```python
from build123d import *

# Parameters (mm, degrees)
F0_W     = 5.75
F0_H     = 3
F2_W     = 8.114334
F2_H     = 7.330208
F3_DEPTH = 3
F4_W     = 7
F4_H     = 3
F5_DEPTH = 18.501


with BuildPart() as f1:
    # F0 (on Top) → F1 (revolve)
    with BuildSketch(Plane.XY):
        with BuildLine():
            Line((4.5, 18.5), (0, 18.5))
            Line((0, 18.5), (0, 6))
            Line((0, 6), (5.75, 6))
            Line((5.75, 6), (5.75, 8))
            add(Edge.make_bspline(
                [(5.75, 8), (5.75, 9.5), (4.5, 10), (4.5, 11.5)],
                knots=[0, 0, 0, 0, 3.716517, 3.716517, 3.716517, 3.716517], degree=3))
            Line((4.5, 11.5), (4.5, 18.5))
        make_face()
        with Locations((2.875, 1.5)):
            Rectangle(F0_W, F0_H)
    revolve(axis=Axis((0, 7.539056, 0), (0, -1, 0)))

    # F2 (on face) → F3 (join, through all)
    with BuildSketch(Plane(origin=(0, 3, 0), x_dir=(-1, 0, 0), z_dir=(0, 1, 0))):
        Rectangle(F2_W, F2_H)
    extrude(amount=F3_DEPTH)

    # F4 (on face) → F5 (cut, through all)
    with BuildSketch(Plane(origin=(0, 18.5, 0), x_dir=(-1, 0, 0), z_dir=(0, 1, 0))):
        Rectangle(F4_W, F4_H)
    extrude(amount=-F5_DEPTH, mode=Mode.SUBTRACT)


solid = f1.part
```
Check sheet for the modelled part. Datum: model origin and axes. Units: mm. A direction names the side the tool comes from. Give positions to 0.01 mm unless a question says otherwise; leave off trailing zeros. Write each loop counter-clockwise with the first axis right and the second up, starting at its lowest first coordinate (ties: lowest second). Pieces come first, ordered by that corner, then holes.
Item 1: Gauge pin test, flat ends, axial feed: pin 1 (2.5 mm diameter, centred on y = 12.5, z = -0.5, fed in from -X); pin 2 (0.9 mm diameter, centred on y = 4, z = -0.5, fed in from -X); pin 3 (5.5 mm diameter, centred on x = 1.5, y = 12.5, fed in from -Z) (3 decimals). Record the tip position at first contact, or that the pin passes through.
Item 2: Cross-section at B-B (y = 13). Enter the section's corners in (x, z).
Item 3: Access from +Z, -Z, +X, -X, +Y, -Y to the whole of each face (thin tool, end or side, straight path). Record for faces 1 (the face through (4.057, 4, 0)), 2 (the face through (-3.5, 9, 0)), 3 (the face through (-0.59, 15.05, 4.46)), 4 (the face through (-4.057, 4, 0)), 5 (the face through (0, 4, -3.665)).
Item 4: Cross-section at A-A (y = 3.5). Enter the section's corners in (x, z).
Item 5: Scan lines: L1, parallel to X at y = 5.75, z = -0.5; L2, parallel to Z at x = 2.25, y = 4; L3, parallel to Y at x = -4.25, z = -1. Record each from-to range of solid material in increasing order.
Item 6: Draft check along Z on faces 6 (the face through (0, 4, 3.665)), 7 (the face through (0, 6, -4)), 8 (the face through (3.5, 9, 0)). Enter one of: released by +Z, released by -Z, zero draft, split by the parting line, or undercut.
Report:
1. pin 1: stops at x = -4.51
1. pin 2: stops at x = -4.06
1. pin 3: stops at z = -5.005
2. outline: circle Ø9 at (0, 0); hole (-3.5, -1.5) - (3.5, -1.5) - (3.5, 1.5) - (-3.5, 1.5) - close
3. face 1: +Z, -Z, +X
3. face 2: +Y, -Y
3. face 3: +Y
3. face 4: +Z, -Z, -X
3. face 5: -Z, +X, -X
4. outline: (-4.06, -3.67) - (4.06, -3.67) - (4.06, 3.67) - (-4.06, 3.67) - close; hole (-3.5, -1.5) - (3.5, -1.5) - (3.5, 1.5) - (-3.5, 1.5) - close
5. L1: x = -4.06 to -3.5, 3.5 to 4.06
5. L2: z = -3.67 to -1.5, 1.5 to 3.67
5. L3: y = 0 to 3, 6 to 18.5
6. face 6: released by +Z
6. face 7: zero draft
6. face 8: undercut
